```python
from build123d import *

# Parameters (mm, degrees)
SKETCH1_W            = 27
SKETCH1_H            = 28
BOSS_EXTRUDE1_DEPTH  = 10
SKETCH2_W            = 20.05
SKETCH2_H            = 10.68
CUT_EXTRUDE1_DEPTH   = 11
M3_CLEARANCE_HOLE1_D = 3.4
M3_CLEARANCE_HOLE2_D = 3.4
CUT_EXTRUDE2_DEPTH   = 2.4
FILLET1_R            = 1
CUT_EXTRUDE8_START   = -2.4
CUT_EXTRUDE8_DEPTH   = 2.4


with BuildPart() as part:
    # Sketch1 → Boss-Extrude1 (new body)
    with BuildSketch(Plane(origin=(0, 0, 0), x_dir=(1, 0, 0), z_dir=(0, 1, 0))):
        with Locations((13.5, 14)):
            Rectangle(SKETCH1_W, SKETCH1_H)
    extrude(amount=BOSS_EXTRUDE1_DEPTH)

    # Sketch2 → Cut-Extrude1 (cut, through all)
    with BuildSketch(Plane(origin=(0, 10, 0), x_dir=(1, 0, 0), z_dir=(0, 1, 0))):
        with Locations((10.025, 14.29)):
            Rectangle(SKETCH2_W, SKETCH2_H)
    extrude(amount=-CUT_EXTRUDE1_DEPTH, mode=Mode.SUBTRACT)

    # M3 Clearance Hole1 (through all)
    with Locations(Plane(origin=(27, 0, 0), x_dir=(0, 0, -1), z_dir=(1, 0, 0))):
        with Locations((14.315, 4.999999998)):
            Hole(M3_CLEARANCE_HOLE1_D / 2)

    # M3 Clearance Hole2 (through all)
    with Locations(Plane(origin=(0, 10, 0), x_dir=(1, 0, 0), z_dir=(0, 1, 0))):
        with Locations((5, 24), (22, 24), (22, 4), (5, 4)):
            Hole(M3_CLEARANCE_HOLE2_D / 2)

    # Sketch7 → Cut-Extrude2 (cut)
    with BuildSketch(Plane(origin=(0, 10, 0), x_dir=(1, 0, 0), z_dir=(0, 1, 0))):
        Polygon((6.58771324, 1.25), (8.175426481, 4), (6.58771324, 6.75), (3.41228676, 6.75), (1.824573519, 4), (3.41228676, 1.25), align=None)
        Polygon((23.58771324, 1.25), (25.175426481, 4), (23.58771324, 6.75), (20.41228676, 6.75), (18.824573519, 4), (20.41228676, 1.25), align=None)
        Polygon((23.58771324, 21.25), (25.175426481, 24), (23.58771324, 26.75), (20.41228676, 26.75), (18.824573519, 24), (20.41228676, 21.25), align=None)
        Polygon((6.58771324, 21.25), (8.175426481, 24), (6.58771324, 26.75), (3.41228676, 26.75), (1.824573519, 24), (3.41228676, 21.25), align=None)
    cut_extrude2 = extrude(amount=-CUT_EXTRUDE2_DEPTH, mode=Mode.SUBTRACT)

    # Mirror1: Cut-Extrude2 across plane
    add(cut_extrude2.mirror(Plane.ZX.offset(5)), mode=Mode.SUBTRACT)

    # Fillet1
    fillet1_edges = [part.edges().sort_by_distance(p)[0] for p in [
        (0, 5, -8.95),
        (0, 5, -19.63),
        (20.05, 5, -19.63),
        (20.05, 5, -8.95),
        (0, 5, -28),
        (27, 5, -28),
        (27, 5, 0),
        (0, 5, 0),
    ]]
    fillet(fillet1_edges, radius=FILLET1_R)

    # Sketch12 → Cut-Extrude8 (cut)
    with BuildSketch(Plane(origin=(27, 0, 0), x_dir=(0, 0, -1), z_dir=(1, 0, 0)).offset(CUT_EXTRUDE8_START)):
        Polygon((14.315, 1.824573517), (17.065, 3.412286757), (17.065, 6.587713238), (14.315, 8.175426478), (11.565, 6.587713238), (11.565, 3.412286757), align=None)
    extrude(amount=CUT_EXTRUDE8_DEPTH, mode=Mode.SUBTRACT)


solid = part.part
```
Geometry check sheet. Reference: the model listing, model coordinates, mm. A direction names the side the tool comes from. Coordinates: 2 decimals unless noted, no trailing zeros. Loops run counter-clockwise (first coordinate to the right, second up) from the corner with the lowest first, then second, coordinate; pieces in that order, holes last. Notation, with made-up numbers: (58, 82.25) - (106, 82.25) arc R20 ccw to (106, 89.25) - close; hole circle Ø7 at (19.25, 67). An arc over 180 degrees is marked (long way). One line per item, written item: value. Start each with the question number.
(1) Cross-section at B-B on y = 5. Enter the section's corners in (x, z) (3 decimals), plus the area to 3 significant figures.
(2) Material ranges on line 1 (Z direction, x = 5, y = 3.6); line 2 (Z direction, x = 22, y = 5.1); line 3 (X direction, y = 6.3, z = -24), recorded low to high. Write a range as [from, to].
(3) Tool access check on faces 4 (the flat face through (25.783, 2.607, -15.671)), 5 (the flat face through (13, 5, 0)), 6 (the flat face through (7.37, 8.817, -2.606)), 7 (the flat face through (22, 1, -6.75)). Record the directions out of +Z, -Z, +X, -X, +Y, -Y that give a thin tool (end or side, any length) a straight path to the whole face; none if there is none.
(4) Depth check by flat-ended pin: P1, Ø4.5, axis at x = 22, z = -24, coming from the -Y side. Enter the tip coordinate at first touch or a pass-through.
(5) Mould release check, pull along X, two halves, no side actions. Record for faces 1 (the cylindrical face through (5.221, 4.964, -25.686)), 2 (the flat face through (0, 5, -4)), 3 (the flat face through (26, 5, -11.565)): released by +X, released by -X, zero draft, split by the parting line, or undercut.
(6) Cross-section at A-A on x = 22. Count the separate pieces of the cut face and the enclosed holes in it, plus the area to 3 significant figures.
(7) Cross-section at D-D on z = -23.5. Enter the section's corners in (x, y), plus the area to 3 significant figures.
Results below:
1. outline: (0, -27) arc R1 ccw to (1, -28) - (26, -28) arc R1 ccw to (27, -27) - (27, -17.065) - (24.6, -17.065) - (24.6, -16.015) - (20.05, -16.015) - (20.05, -18.63) arc R1 cw to (19.05, -19.63) - (1, -19.63) arc R1 ccw to (0, -20.63) - close; (0, -7.95) arc R1 ccw to (1, -8.95) - (19.05, -8.95) arc R1 cw to (20.05, -9.95) - (20.05, -12.615) - (24.6, -12.615) - (24.6, -11.565) - (27, -11.565) - (27, -1) arc R1 ccw to (26, 0) - (1, 0) arc R1 ccw to (0, -1) - close; hole circle Ø3.4 at (5, -24); hole circle Ø3.4 at (5, -4); hole circle Ø3.4 at (22, -24); hole circle Ø3.4 at (22, -4)
1. area: 476 mm2
2. line 1: z = [-28, -25.7], [-22.3, -19.63], [-8.95, -5.7], [-2.3, 0]
2. line 2: z = [-28, -25.7], [-22.3, -16.01], [-12.62, -5.7], [-2.3, 0]
2. line 3: x = [0, 3.3], [6.7, 20.3], [23.7, 27]
3. face 4: +X
3. face 5: +Z, +X, -X, +Y, -Y
3. face 6: +Y
3. face 7: -Y
4. P1: stops at y = 2.4
5. face 1: undercut
5. face 2: released by -X
5. face 3: zero draft
6. separate pieces: 3
6. enclosed holes: 1
6. area: 183 mm2
7. outline: (0, 0) - (2.11, 0) - (2.11, 2.4) - (3.38, 2.4) - (3.38, 7.6) - (2.11, 7.6) - (2.11, 10) - (0, 10) - close; (6.62, 2.4) - (7.89, 2.4) - (7.89, 0) - (19.11, 0) - (19.11, 2.4) - (20.38, 2.4) - (20.38, 7.6) - (19.11, 7.6) - (19.11, 10) - (7.89, 10) - (7.89, 7.6) - (6.62, 7.6) - close; (23.62, 2.4) - (24.89, 2.4) - (24.89, 0) - (27, 0) - (27, 10) - (24.89, 10) - (24.89, 7.6) - (23.62, 7.6) - close
7. area: 181 mm2
